Build history of the part. All positions in model axes, mm. Face numbers are marked on the shaded views. Coordinates: 2 decimals unless noted, no trailing zeros. Order: outer loops, then holes, each group sorted by start corner. A loop starts at its lowest first (then second) coordinate and runs counter-clockwise, first axis right, second up. Notation, with made-up numbers: (-16.75, 73.25) -> (-11.75, 73.25) arc R29 cw to (-11.75, 103.25) -> close; hole circle Ø7 at (44.25, -28.5). An arc over 180 degrees is marked (long way). Write each question's results on one line, items separated by ' | '.
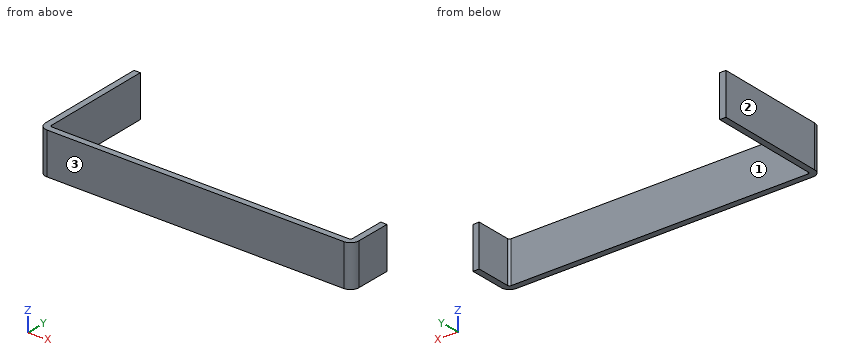
Autodesk Inventor part; units mm, degrees
ref_plane "YZ Plane" through (0, 0, 0) normal (1, 0, 0) x (0, 1, 0)
ref_plane "XZ Plane" through (0, 0, 0) normal (0, 1, 0) x (-1, 0, 0)
ref_plane "XY Plane" through (0, 0, 0) normal (0, 0, 1) x (1, 0, 0)
sketch "Sketch1" plane through (0, 0, 0) normal (0, 0, 1) x (1, 0, 0)
  line L0 (0, 138) -> (0, -23) construction
  line L1 (-361.2743, 0) -> (60.6456, 0) construction
  line L2 (0, 0) -> (0.3713, 41.5996)
  line L3 (0.3713, 41.5996) -> (-5.6284, 41.6531)
  line L4 (-5.6284, 41.6531) -> (-5.9467, 6)
  line L5 (-5.9467, 6) -> (-295, 6)
  line L6 (-295, 6) -> (-295, 115)
  line L7 (-295, 115) -> (-301, 115)
  line L8 (-301, 115) -> (-301, 0)
  line L9 (0, 0) -> (-301, 0)
  dimension "d4" = 41.5996
  dimension "d5" = 301
  dimension "d6" = 115
  dimension "d7" = 6
  dimension "d8" = 6
  dimension "d9" = 6
extrude "Extrusion3" add sketch "Sketch1" along normal blind 40
fillet "Fillet1" radius 2 2 edges at (-5.9467, 6, 20) (-295, 6, 20)
fillet "Fillet2" radius 8 2 edges at (0, 0, 20) (-301, 0, 20)
equation "\"d8\" = d7"
equation "\"d9\" = d7"
properties part number "17-0028-0119" material "Copper"
Item 1: Slice it at C-C, the plane x = -224. List the corners of the cut face in (y, z).
Answer:
outline: (0, 0) -> (6, 0) -> (6, 40) -> (0, 40) -> close
Item 2: Slice it at D-D, the plane y = 97. List the corners of the cut face in (x, z).
Answer:
outline: (-301, 0) -> (-295, 0) -> (-295, 40) -> (-301, 40) -> close
Item 3: Drill centre lines: line 1 (X direction, y = 10, z = 10); line 2 (Y direction, x = -167.5, z = 4.5); line 3 (X direction, y = 82.5, z = 8.5). Where is each one in solid material? Low to high. Write a range as from..to.
Answer:
line 1: x = -301..-295, -5.91..0.09 | line 2: y = 0..6 | line 3: x = -301..-295
Item 4: Pin check, flat tips, straight feed: pin 1 (2 mm diameter, centred on x = -259.5, z = 34, fed in from +Y); pin 2 (12 mm diameter, centred on y = 79.5, z = 28.5, fed in from +X). Stop position of each tip, or through.
Answer:
pin 1: stops at y = 6 | pin 2: stops at x = -295
Item 5: Slice it at B-B, the plane z = 28. List the corners of the cut face in (x, y).
Answer:
outline: (-301, 8) arc R8 ccw to (-293, 0) -> (-7.93, 0) arc R8 ccw to (0.07, 7.93) -> (0.37, 41.6) -> (-5.63, 41.65) -> (-5.93, 7.98) arc R2 cw to (-7.93, 6) -> (-293, 6) arc R2 cw to (-295, 8) -> (-295, 115) -> (-301, 115) -> close
Item 6: Pull direction X, two halves, no side cores. Call the marked faces 1, 2 and 3: released by +X, released by -X, zero draft, split by the parting line, or undercut.
Answer:
face 1: undercut | face 2: released by -X | face 3: zero draft
Item 7: Slice it at A-A, the plane y = 20. List the corners of the cut face in (x, z), and give its area (3 significant figures).
Answer:
outline: (-301, 0) -> (-295, 0) -> (-295, 40) -> (-301, 40) -> close; (-5.82, 0) -> (0.18, 0) -> (0.18, 40) -> (-5.82, 40) -> close | area: 480 mm^2
